from build123d import *

# Parameters (mm, degrees)
SKETCH1_R           = 40
BOSS_EXTRUDE1_DEPTH = 90
SKETCH2_R           = 35
CUT_EXTRUDE1_DEPTH  = 85
FILLET1_R           = 2
FILLET2_R           = 2
FILLET4_R           = 5


with BuildPart() as part:
    # Sketch1 → Boss-Extrude1 (new body)
    with BuildSketch(Plane(origin=(0, 0, 0), x_dir=(1, 0, 0), z_dir=(0, 1, 0))):
        Circle(SKETCH1_R)
    extrude(amount=BOSS_EXTRUDE1_DEPTH)

    # Sketch2 → Cut-Extrude1 (cut)
    with BuildSketch(Plane(origin=(0, 90, 0), x_dir=(1, 0, 0), z_dir=(0, 1, 0))):
        Circle(SKETCH2_R)
    extrude(amount=-CUT_EXTRUDE1_DEPTH, mode=Mode.SUBTRACT)

    # Fillet1
    fillet1_edges = [part.edges().sort_by_distance(p)[0] for p in [
        (-40, 90, 0),
    ]]
    fillet(fillet1_edges, radius=FILLET1_R)

    # Fillet2
    fillet2_edges = [part.edges().sort_by_distance(p)[0] for p in [
        (-35, 90, 0),
    ]]
    fillet(fillet2_edges, radius=FILLET2_R)

    # Fillet4
    fillet4_edges = [part.edges().sort_by_distance(p)[0] for p in [
        (-35, 5, 0),
    ]]
    fillet(fillet4_edges, radius=FILLET4_R)


solid = part.part
Source: CAD feature listing. Evaluate the final solid. Frame: model axes, mm. A direction names the side the tool comes from. Give positions to 0.01 mm unless a question says otherwise; leave off trailing zeros. Write each loop counter-clockwise with the first axis right and the second up, starting at its lowest first coordinate (ties: lowest second). Pieces come first, ordered by that corner, then holes. Notation, with made-up numbers: (-34.75, 15.25) -> (-15.75, 15.25) arc R10 cw to (-15.75, 31.25) -> close; hole circle Ø3 at (78.5, 79). An arc over 180 degrees is marked (long way). Return JSON: item names as keys, results as strings. Group by question number.
1. Access query for faces 1 (the face through (0, 5, 0)), 2 (the face through (-1, 0, -1)). Directions: +Z, -Z, +X, -X, +Y, -Y. A direction counts if a zero-diameter tool reaches every point of the face in a straight line with its end or side. Return the directions, or none.
2. Section B-B, the plane x = 0. Output: boundary loops of the cut face in (y, z), then the cut area to 3 significant figures.
3. Pin query (flat end, axial travel): pin 1 Ø2 at (x, y) = (2.5, 53.5) entering from -Z; pin 2 Ø10 at (y, z) = (38, -9) entering from +X; pin 3 Ø4 at (x, y) = (-13.5, 61.5) entering from -Z. Return the tip coordinate at first contact, or that it passes through.
4. Section C-C, the plane y = 27. Output: boundary loops of the cut face in (x, z).
5. Mould query, pull axis X, two halves, no side actions, for faces 3 (the face through (-8.67, 43.38, 39.05)), 4 (the face through (-28, 50, 21)), 5 (the face through (8.3, 90, 36.4)). Classes: +X half, -X half, draft (parallel to the pull), parting line (faces both ways), or undercut.
6. Material intervals for line 1 (Z direction, x = 0, y = 61.5); line 2 (Z direction, x = -32, y = 11), sorted ascending. Write a range as from..to.
7. Section A-A, the plane z = 0. Output: boundary loops of the cut face in (x, y).
Determined:
{
 "1": {"face 1": "+Y", "face 2": "+Z, -Z, +X, -X, -Y"},
 "2": {"outline": "(0, -40) -> (88, -40) arc R2 ccw to (90, -38) -> (90, -37) arc R2 ccw to (88, -35) -> (10, -35) arc R5 cw to (5, -30) -> (5, 30) arc R5 cw to (10, 35) -> (88, 35) arc R2 ccw to (90, 37) -> (90, 38) arc R2 ccw to (88, 40) -> (0, 40) -> close", "area": "1,260 mm2"},
 "3": {"pin 1": "stops at z = -39.97", "pin 2": "stops at x = 39.8", "pin 3": "stops at z = -38.31"},
 "4": {"outline": "circle Ø80 at (0, 0); hole circle Ø70 at (0, 0)"},
 "5": {"face 3": "parting line", "face 4": "undercut", "face 5": "draft"},
 "6": {"line 1": "z = -40..-35, 35..40", "line 2": "z = -24..-14.18, 14.18..24"},
 "7": {"outline": "(-40, 0) -> (40, 0) -> (40, 88) arc R2 ccw to (38, 90) -> (37, 90) arc R2 ccw to (35, 88) -> (35, 10) arc R5 cw to (30, 5) -> (-30, 5) arc R5 cw to (-35, 10) -> (-35, 88) arc R2 ccw to (-37, 90) -> (-38, 90) arc R2 ccw to (-40, 88) -> close"}
}
